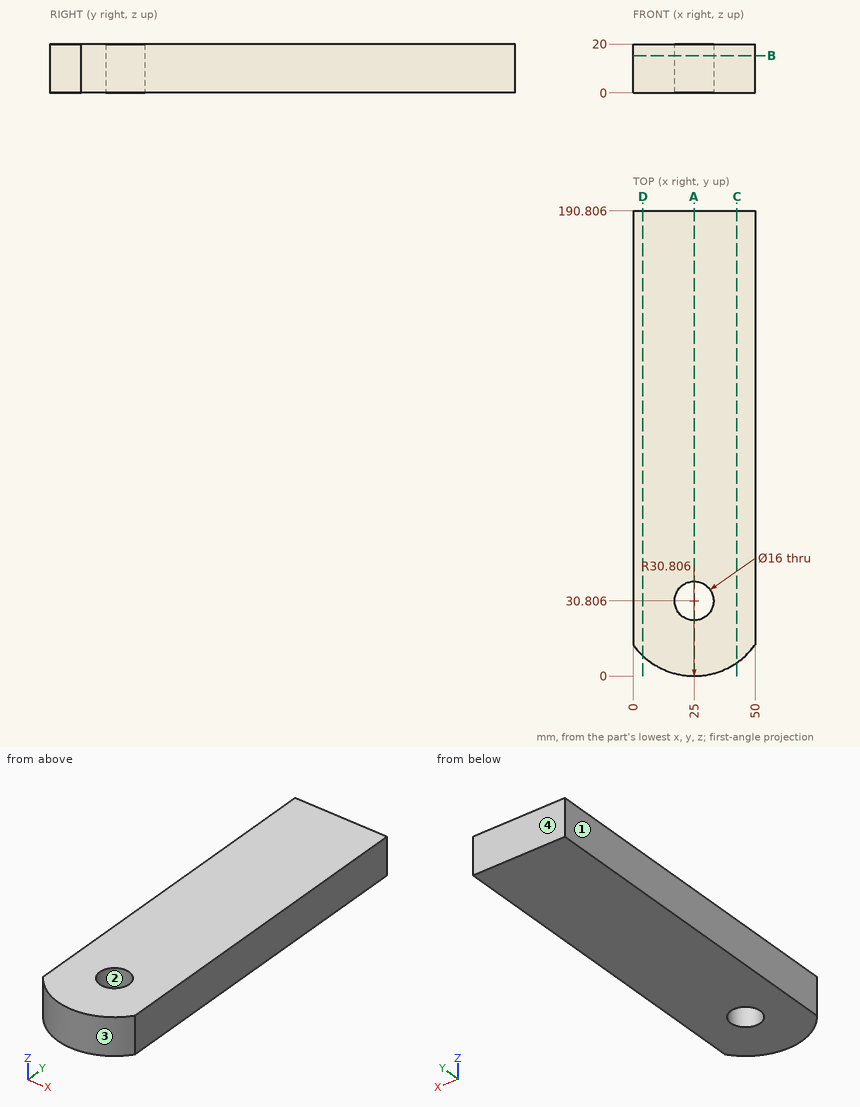
Print and shaded views of the part. All mm, measured from the part's lowest x, y and z. Coordinates: 2 decimals unless noted, no trailing zeros. Write each loop counter-clockwise with the first axis right and the second up, starting at its lowest first coordinate (ties: lowest second). Pieces come first, ordered by that corner, then holes.
(1) Cut at D-D, the plane x = 4. List the corners of the cut face in (y, z), and give its area (3 significant figures).
(2) Cut at C-C, the plane x = 42.5. List the corners of the cut face in (y, z).
(3) Cut at A-A, the plane x = 25. List the corners of the cut face in (y, z), and give its area (3 significant figures).
(4) Cut at B-B, the plane z = 15.25. List the corners of the cut face in (x, y), and give its area (3 significant figures).
(5) Drill centre lines: probe 1 along Y at (x, z) = (25.5, 14.5); probe 2 along Y at (x, z) = (23, 13) (1 decimal); probe 3 along Y at (x, z) = (5, 19) (1 decimal). Where is each one in solid material? Low to high.
(6) Two-plate mould, pull along Y, no slides. Class the marked faces 1, 2, 3 and 4: +Y half, -Y half, draft (parallel to the pull), parting line (faces both ways), or undercut.
(7) Flat gauge pins, fed straight in: pin 1 (8 mm diameter, centred on x = 9.5, z = 16.5, fed in from -Y); pin 2 (10 mm diameter, centred on x = 39.5, z = 3, fed in from -Y); pin 3 (5 mm diameter, centred on x = 19.5, z = 14.5, fed in from -Y). Where does each tip first touch, or does it go through?
Geometry says:
1. outline: (8.27, 0) - (190.81, 0) - (190.81, 20) - (8.27, 20) - close
1. area: 3,650 mm2
2. outline: (5.45, 0) - (190.81, 0) - (190.81, 20) - (5.45, 20) - close
3. outline: (0, 0) - (22.81, 0) - (22.81, 20) - (0, 20) - close; (38.81, 0) - (190.81, 0) - (190.81, 20) - (38.81, 20) - close
3. area: 3,500 mm2
4. outline: (0, 12.81) arc R30.81 ccw to (50, 12.81) - (50, 190.81) - (0, 190.81) - close; hole circle Ø16 at (25, 30.81)
4. area: 9,150 mm2
5. probe 1: y = 0 to 22.82, 38.79 to 190.81
5. probe 2: y = 0.1 to 23.1, 38.6 to 190.8
5. probe 3: y = 7.4 to 190.8
6. face 1: draft
6. face 2: undercut
6. face 3: -Y half
6. face 4: +Y half
7. pin 1: stops at y = 2.23
7. pin 2: stops at y = 1.5
7. pin 3: stops at y = 0.15
